from build123d import *

# Parameters (mm, degrees)
ESTRUSIONE_ESTRUSIONE1_DEPTH                         = 18
TAGLIO_ESTRUSIONE1_DEPTH                             = 78.129760793
TAGLIO_ESTRUSIONE1_DEPTH_BACK                        = 78.129760793
SCHIZZO2_W                                           = 3
SCHIZZO2_H                                           = 42
FORO_8_0_8_1_D                                       = 8
FORO_5_0_5_2_D                                       = 5
FORO_LAMATO_PER_VITE_M6_A_TESTA_CILINDRI_D           = 6.6
FORO_LAMATO_PER_VITE_M6_A_TESTA_CILINDRI_CBORE_D     = 11
FORO_LAMATO_PER_VITE_M6_A_TESTA_CILINDRI_CBORE_DEPTH = 6.4
FORO_5_0_5_3_AT_2_COUNT                              = 2
FORO_5_0_5_3_AT_2_PITCH                              = 26.305892876
SMUSSO1_SIZE                                         = 3
RACCORDO1_R                                          = 0.2


with BuildPart() as part:
    # Schizzo1 → Estrusione-Estrusione1 (new body)
    with BuildSketch(Plane.XY):
        Polygon((-60, 45), (60, 45), (60, 19), (45, 19), (45, -19), (60, -19), (60, -45), (-60, -45), (-60, -19), (-45, -19), (-45, 19), (-60, 19), align=None)
    extrude(amount=ESTRUSIONE_ESTRUSIONE1_DEPTH)

    # Schizzo2 → Taglio-Estrusione1 (cut, two sides: drawn at the far end of the back side and taken through both)
    with BuildSketch(Plane(origin=(0, 0, 0), x_dir=(0, 0, -1), z_dir=(1, 0, 0)).offset(-TAGLIO_ESTRUSIONE1_DEPTH_BACK)):
        with Locations((-1.5, 0)):
            Rectangle(SCHIZZO2_W, SCHIZZO2_H)
    extrude(amount=TAGLIO_ESTRUSIONE1_DEPTH + TAGLIO_ESTRUSIONE1_DEPTH_BACK, mode=Mode.SUBTRACT)

    # Schizzo4 → Foro filettato M6-1 (revolve, cut)
    with BuildSketch(Plane(origin=(45, 0, 10.5), x_dir=(0, 0, -1), z_dir=(0, 1, 0))):
        Polygon((0, 0), (0, 21.502151548), (2.5, 20), (2.5, 0), align=None)
    foro_filettato_m6_1 = revolve(axis=Axis((51.35, 0, 10.5), (-1, 0, 0)), mode=Mode.SUBTRACT)

    # Foro Ø8.0 (8)-1 (through all)
    with Locations(Plane.XY.offset(18)):
        with Locations((0, 0)):
            Hole(FORO_8_0_8_1_D / 2)

    # Foro Ø5.0 (5)-2 (through all)
    with Locations(Plane.XY.offset(18)):
        with Locations((20, -10), (-20, 10)):
            Hole(FORO_5_0_5_2_D / 2)

    # Foro lamato per Vite M6 a testa cilindrica-1 (through all)
    with Locations(Plane(origin=(0, 0, 3), x_dir=(-1, 0, 0), z_dir=(0, 0, -1))):
        with Locations((-20, 10), (20, -10)):
            CounterBoreHole(FORO_LAMATO_PER_VITE_M6_A_TESTA_CILINDRI_D / 2, FORO_LAMATO_PER_VITE_M6_A_TESTA_CILINDRI_CBORE_D / 2, FORO_LAMATO_PER_VITE_M6_A_TESTA_CILINDRI_CBORE_DEPTH)

    # Schizzo14 → Foro Ø5.0 (5)-3 (revolve, cut)
    with BuildSketch(Plane(origin=(45, -13, 12.5), x_dir=(0, 0, -1), z_dir=(0, 1, 0))):
        Polygon((0, 0), (0, 11.502151548), (2.5, 10), (2.5, 0), align=None)
    foro_5_0_5_3 = revolve(axis=Axis((51.35, -13, 12.5), (-1, 0, 0)), mode=Mode.SUBTRACT)

    # Foro Ø5.0 (5)-3 at 2: Foro Ø5.0 (5)-3 ×2
    with Locations(*[Vector(0, 0.9883716976506173, -0.15205718425394077) * (i * FORO_5_0_5_3_AT_2_PITCH) for i in range(1, FORO_5_0_5_3_AT_2_COUNT)]):
        add(foro_5_0_5_3, mode=Mode.SUBTRACT)

    # Smusso1
    smusso1_edges = [part.edges().sort_by_distance(p)[0] for p in [
        (0, 45, 18),
        (0, -45, 18),
    ]]
    chamfer(smusso1_edges, length=SMUSSO1_SIZE)

    # Raccordo1
    raccordo1_edges = [part.edges().sort_by_distance(p)[0] for p in [
        (45, -19, 10.5),
        (45, 19, 10.5),
        (-45, 19, 10.5),
        (-45, -19, 10.5),
        (0, -21, 3),
        (0, 21, 3),
    ]]
    fillet(raccordo1_edges, radius=RACCORDO1_R)

    # Specchia1: Foro filettato M6-1, Foro Ø5.0 (5)-3 across plane
    add(foro_filettato_m6_1.mirror(Plane(origin=(0, 0, 0), x_dir=(0, 0, 1), z_dir=(1, 0, 0))), mode=Mode.SUBTRACT)
    add(foro_5_0_5_3.mirror(Plane(origin=(0, 0, 0), x_dir=(0, 0, 1), z_dir=(1, 0, 0))), mode=Mode.SUBTRACT)

    # Specchia1 copy 1 sketch → Specchia1 copy 1 (revolve, cut)
    with BuildSketch(Plane(origin=(-45, 13, 8.5), x_dir=(0, 0, -1), z_dir=(0, 1, 0))):
        Polygon((0, 0), (0, -11.502151548), (2.5, -10), (2.5, 0), align=None)
    revolve(axis=Axis((-51.35, 13, 8.5), (-1, 0, 0)), mode=Mode.SUBTRACT)


solid = part.part
The listing builds one solid part. Answer for the finished solid, in the listing's coordinates (mm). A direction names the side the tool comes from. Give positions to 0.01 mm unless a question says otherwise; leave off trailing zeros. Write each loop counter-clockwise with the first axis right and the second up, starting at its lowest first coordinate (ties: lowest second). Pieces come first, ordered by that corner, then holes. Notation, with made-up numbers: (82, 60) - (110, 60) arc R24 cw to (110, 83) - close; hole circle Ø10 at (7.25, 56.25). An arc over 180 degrees is marked (long way). Use a Markdown table: item, result.
1. A tool of negligible diameter and unlimited length cuts with its end or side. For faces 4 (the flat face through (52, -19, 10)), 5 (the cylindrical face through (-35, 0, 13)), 6 (the flat face through (-45, 0, 7)), from which of +Z, -Z, +X, -X, +Y, -Y can it reach the whole face along a straight path? Write none if from no direction.
Values follow:
| item | result |
|---|---|
| face 4 | +Z, -Z, +X |
| face 5 | -X |
| face 6 | +Z, -Z, -X |
2. Each of these flat-tipped pins is pushed along its axis until it touches: P1, Ø6.5, axis at y = 13, z = 8.5, coming from the -X side; P2, Ø9, axis at x = 19.5, y = 10, coming from the -Z side; P3, Ø6, axis at x = -47.5, y = -6.5, coming from the -Z side; P4, Ø5, axis at x = 0, y = 0, coming from the -Z side. Where does it stop, or does it pass through?
Values follow:
| item | result |
|---|---|
| P1 | stops at x = -45 |
| P2 | stops at z = 9.4 |
| P3 | stops at z = 3 |
| P4 | passes through |
3. Find the intervals of material crossed by probe 1 along Y at (x, z) = (20, 7.75); probe 2 along Y at (x, z) = (-20, 5.25); probe 3 along Y at (x, z) = (12, 2.75), in increasing order. Write a range as from..to.
Values follow:
| item | result |
|---|---|
| probe 1 | y = -45..-12.5, -7.5..4.5, 15.5..45 |
| probe 2 | y = -45..-15.5, -4.5..7.5, 12.5..45 |
| probe 3 | y = -45..-21, 21..45 |
4. Section B-B on z = 1.5 is taken. Write down the section's boundary in (x, y), plus the area to 3 significant figures.
Values follow:
| item | result |
|---|---|
| outline | (-60, -45) - (60, -45) - (60, -21) - (-60, -21) - close; (-60, 21) - (60, 21) - (60, 45) - (-60, 45) - close |
| area | 5,760 mm² |
5. Section A-A on x = 0 is taken. Write down the section's boundary in (y, z), plus the area to 3 significant figures.
Values follow:
| item | result |
|---|---|
| outline | (-45, 0) - (-21, 0) - (-21, 2.8) arc R0.2 cw to (-20.8, 3) - (-4, 3) - (-4, 18) - (-42, 18) - (-45, 15) - close; (4, 3) - (20.8, 3) arc R0.2 cw to (21, 2.8) - (21, 0) - (45, 0) - (45, 15) - (42, 18) - (4, 18) - close |
| area | 1,370 mm² |
6. For a pull along X with two mould halves and no side action, classify faces 1 (the cylindrical face through (0.867, -3.905, 10.395)), 2 (the flat face through (-1, 21, 1)), 3 (the conical face through (33.759, 13.264, 8.845)) as released by +X, released by -X, zero draft, split by the parting line, or undercut.
Values follow:
| item | result |
|---|---|
| face 1 | undercut |
| face 2 | zero draft |
| face 3 | released by +X |
